Input: part model. Units: mm. Frame: model coordinates. Face numbers are marked on the shaded views. A direction names the side the tool comes from. Round coordinates to 2 decimals unless told otherwise and drop trailing zeros. Loops run counter-clockwise (first coordinate to the right, second up) from the corner with the lowest first, then second, coordinate; pieces in that order, holes last. Notation, with made-up numbers: M 18.5,26 L 28.5,26 A19 cw 28.5,61 Z; hole C 48,13 d5. An arc over 180 degrees is marked long. Put each result on its own line as item: value. Start each with the question number.
1) Pin query (flat end, axial travel): pin 1 (2 mm diameter, centred on y = 17, z = 15.5, fed in from +X); pin 2 (5 mm diameter, centred on x = 153, y = -7, fed in from +Z); pin 3 (4 mm diameter, centred on x = 199.5, z = 6, fed in from -Y); pin 4 (2 mm diameter, centred on x = 82, y = -2.5, fed in from -Z). Return the tip coordinate at first contact, or that it passes through.
2) Section C-C on y = 10.5. Output: boundary loops of the cut face in (x, z), plus the area to 3 significant figures.
3) Draft query along Y for the marked faces 3 and 4. Return one class per face: +Y half, -Y half, draft (parallel to the pull), parting line (faces both ways), or undercut.
4) Line query: probe 1 along X at (y, z) = (4, 4); probe 2 along Y at (x, z) = (153, 2.5); probe 3 along Y at (x, z) = (-0.95, 8.75). Output: solid intervals per line, ascending.
5) Section A-A on z = 13. Output: boundary loops of the cut face in (x, y), plus the area to 3 significant figures.
6) Section B-B on x = 214. Output: boundary loops of the cut face in (y, z), plus the area to 3 significant figures.
7) Reachability of the marked faces 1 and 2 from +Z, -Z, +X, -X, +Y, -Y: full face, straight path, thin tool, end or side. Return the list, or none.
from build123d import *

# Parameters (mm, degrees)
SKETCH1_W           = 250
SKETCH1_H           = 5
SKETCH1_W_2         = 143
SKETCH1_W_3         = 87
BOSS_EXTRUDE1_DEPTH = 17.5
SKETCH1_3_W         = 250
SKETCH1_3_H         = 5
CUT_EXTRUDE1_DEPTH  = 8.5
SKETCH2_R           = 2
CUT_EXTRUDE2_DEPTH  = 8.5
SKETCH1_5_R         = 2
BOSS_EXTRUDE2_DEPTH = 8.5
BOSS_EXTRUDE3_DEPTH = 30


with BuildPart() as part:
    # Sketch1 → Boss-Extrude1 (new body)
    with BuildSketch(Plane.XY):
        with Locations((125, 2.5)):
            Rectangle(SKETCH1_W, SKETCH1_H)
        Polygon((249, 8), (250, 7), (250, 5), (0, 5), (0, 8), align=None)
        Polygon((0, 23.5), (0, 8), (0, 5), (0, 0), (-3, 0), (-3, 23.5), align=None)
        with Locations((71.5, 2.5)):
            Rectangle(SKETCH1_W_2, SKETCH1_H)
        with Locations((206.5, 2.5)):
            Rectangle(SKETCH1_W_3, SKETCH1_H)
    extrude(amount=BOSS_EXTRUDE1_DEPTH)

    # Sketch1_3 → Cut-Extrude1 (cut)
    with BuildSketch(Plane.XY):
        with Locations((125, 2.5)):
            Rectangle(SKETCH1_3_W, SKETCH1_3_H)
    extrude(amount=CUT_EXTRUDE1_DEPTH, mode=Mode.SUBTRACT)

    # Sketch2 → Cut-Extrude2 (cut)
    with BuildSketch(Plane(origin=(0, 0, 0), x_dir=(0, 0, -1), z_dir=(1, 0, 0))):
        with Locations((-8.75, 15.75)):
            Circle(SKETCH2_R)
    extrude(amount=-CUT_EXTRUDE2_DEPTH, mode=Mode.SUBTRACT)

    # Sketch1_5 → Boss-Extrude2 (add)
    with BuildSketch(Plane.XY):
        with BuildLine():
            Line((163, 5), (143, 5))
            Line((143, 5), (143, -7))
            ThreePointArc((143, -7), (153, -17), (163, -7))
            Line((163, -7), (163, 5))
        make_face()
        with Locations((153, -7)):
            Circle(SKETCH1_5_R, mode=Mode.SUBTRACT)
    extrude(amount=BOSS_EXTRUDE2_DEPTH)

    # Sketch4 → Boss-Extrude3 (add)
    with BuildSketch(Plane(origin=(250, 0, 0), x_dir=(0, 0, -1), z_dir=(1, 0, 0))):
        Polygon((-5.029428908, -6.92820323), (-9.029428908, 0), (-17.029428908, 0), (-21.029428908, -6.92820323), (-17.029428908, -13.856406461), (-9.029428908, -13.856406461), align=None)
    extrude(amount=-BOSS_EXTRUDE3_DEPTH)


solid = part.part
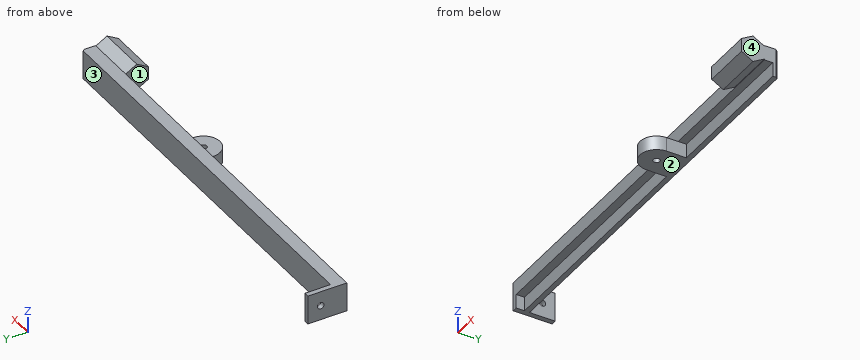
Geometry results:
1. pin 1: stops at x = 0
1. pin 2: stops at z = 8.5
1. pin 3: stops at y = 5
1. pin 4: passes through
2. outline: M -3,0 L 0,0 L 0,17.5 L -3,17.5 Z
2. area: 52.5 mm²
3. face 3: +Y half
3. face 4: draft
4. probe 1: x = -3 to 0, 143 to 163
4. probe 2: y = -17 to -9, -5 to 8
4. probe 3: y = 0 to 13.75, 17.75 to 23.5
5. outline: M -3,0 L 220,0 L 220,-13.86 L 250,-13.86 L 250,7 L 249,8 L 0,8 L 0,23.5 L -3,23.5 Z
5. area: 2,490 mm²
6. outline: M 0,8.5 L 5,8.5 L 5,0 L 8,0 L 8,17.5 L 0,17.5 Z
6. area: 97.5 mm²
7. face 1: +Z, -Z, -Y
7. face 2: -Z, +X, -X, +Y, -Y
